Geometry: final body of the model. Coordinates: model frame, mm. A direction names the side the tool comes from. Round coordinates to 2 decimals unless told otherwise and drop trailing zeros. Write each loop counter-clockwise with the first axis right and the second up, starting at its lowest first coordinate (ties: lowest second). Pieces come first, ordered by that corner, then holes. Notation, with made-up numbers: (47, -34.5) -> (99, -34.5) arc R17 cw to (99, -22.5) -> close; hole circle Ø1 at (32, 86). An arc over 180 degrees is marked (long way). Use one line per item in the form item = value. Start each with the question number.
1. Cut plane D-D, the plane y = 4.75. Return the cut outline in (x, z), plus the area to 3 significant figures.
2. Draft query along Z for faces 1 (the face through (-61, 20, 34.421)), 2 (the face through (-50.91, 3.04, 53.85)), 3 (the face through (-47.459, 3, 45)). Return one class per face: pulls with the +Z half, pulls with the -Z half, needs draft (parallel to the pull), parting line crosses it, or undercut.
3. Cut plane A-A, the plane y = 16.5. Return the cut outline in (x, z), plus the area to 3 significant figures.
4. Pin query (flat end, axial travel): pin 1 Ø5 at (x, z) = (-70.5, 39) entering from +Y; pin 2 Ø10 at (y, z) = (16, 50) entering from -X; pin 3 Ø10 at (y, z) = (18.5, 50) entering from +X. Return the tip coordinate at first contact, or that it passes through.
5. Line query: L1, parallel to Z at x = -70, y = 1; L2, parallel to X at y = 15.5, z = 41; L3, parallel to Y at x = -59.5, z = 52.25. Output: solid intervals per line, ascending.
6. Reachability of faces 4 (the face through (-53.459, 15, 45)), 5 (the face through (-70.79, 3.04, 53.11)), 6 (the face through (-60, 12, 46)), 7 (the face through (-66.459, 15, 45)) from +Z, -Z, +X, -X, +Y, -Y: full face, straight path, thin tool, end or side. Return the list, or none.
7. Cut plane B-B, the plane z = 42.75. Return the cut outline in (x, y).
8. Cut plane C-C, the plane x = -61.25. Return the cut outline in (y, z), plus the area to 3 significant figures.
```python
from build123d import *

# Parameters (mm, degrees)
SKETCH_1_W          = 25
SKETCH_1_H          = 25
EXTRUDE_1_DEPTH     = 23
SKETCH_2_W          = 6
SKETCH_2_H          = 25
CUT_EXTRUDE_1_DEPTH = 17
SKETCH_3_R          = 1.5
CUT_EXTRUDE_2_DEPTH = 6
SKETCH_7_W          = 9
SKETCH_7_H          = 9
CUT_EXTRUDE_3_DEPTH = 23
SKETCH_8_R          = 3.1
CUT_EXTRUDE_4_DEPTH = 23


with BuildPart() as part:
    # 草图1 → 凸台-拉伸1 (new body)
    with BuildSketch(Plane(origin=(0, 0, 0), x_dir=(1, 0, 0), z_dir=(0, 1, 0))):
        with Locations((-59.958661712, -44.921006296)):
            Rectangle(SKETCH_1_W, SKETCH_1_H)
    extrude(amount=EXTRUDE_1_DEPTH)

    # 草图2 → 切除-拉伸1 (cut)
    with BuildSketch(Plane(origin=(0, 23, 0), x_dir=(1, 0, 0), z_dir=(0, 1, 0))):
        with Locations((-69.458661712, -44.921006296)):
            Rectangle(SKETCH_2_W, SKETCH_2_H)
        with Locations((-50.458661712, -44.921006296)):
            Rectangle(SKETCH_2_W, SKETCH_2_H)
    extrude(amount=-CUT_EXTRUDE_1_DEPTH, mode=Mode.SUBTRACT)

    # 草图3 → 切除-拉伸2 (cut)
    with BuildSketch(Plane(origin=(0, 6, 0), x_dir=(1, 0, 0), z_dir=(0, 1, 0))):
        with Locations(Location((-69.458661712, -37.421006296, 0), (0, 0, 270))):
            Circle(SKETCH_3_R)
        with Locations(Location((-69.458661712, -52.421006296, 0), (0, 0, 270))):
            Circle(SKETCH_3_R)
    cut_extrude_2 = extrude(amount=-CUT_EXTRUDE_2_DEPTH, mode=Mode.SUBTRACT)

    # 镜向1: 切除-拉伸2 across plane
    add(cut_extrude_2.mirror(Plane.ZY.offset(59.958661712)), mode=Mode.SUBTRACT)

    # 草图7 → 切除-拉伸3 (cut)
    with BuildSketch(Plane.XY.offset(57.421006296)):
        with Locations((-59.958661712, 16.5)):
            Rectangle(SKETCH_7_W, SKETCH_7_H)
    extrude(amount=-CUT_EXTRUDE_3_DEPTH, mode=Mode.SUBTRACT)

    # 草图8 → 切除-拉伸4 (cut)
    with BuildSketch(Plane.XY.offset(34.421006296)):
        with Locations((-59.958661712, 16.5)):
            Circle(SKETCH_8_R)
    extrude(amount=-CUT_EXTRUDE_4_DEPTH, mode=Mode.SUBTRACT)


solid = part.part
```
Outcome:
q1.outline = (-72.46, 32.42) -> (-47.46, 32.42) -> (-47.46, 57.42) -> (-72.46, 57.42) -> close; hole circle Ø3 at (-69.46, 37.42); hole circle Ø3 at (-69.46, 52.42); hole circle Ø3 at (-50.46, 37.42); hole circle Ø3 at (-50.46, 52.42)
q1.area = 597 mm^2
q2.face_1 = pulls with the +Z half
q2.face_2 = undercut
q2.face_3 = needs draft
q3.outline = (-66.46, 32.42) -> (-63.06, 32.42) -> (-63.06, 34.42) -> (-64.46, 34.42) -> (-64.46, 57.42) -> (-66.46, 57.42) -> close; (-56.86, 32.42) -> (-53.46, 32.42) -> (-53.46, 57.42) -> (-55.46, 57.42) -> (-55.46, 34.42) -> (-56.86, 34.42) -> close
q3.area = 106 mm^2
q4.pin_1 = 6
q4.pin_2 = -66.46
q4.pin_3 = -53.46
q5.L1 = 32.42 to 36.02, 38.82 to 51.02, 53.82 to 57.42
q5.L2 = -66.46 to -64.46, -55.46 to -53.46
q5.L3 = 0 to 12, 21 to 23
q6.face_4 = +Z, -Z, +X, +Y
q6.face_5 = +Y, -Y
q6.face_6 = +Z
q6.face_7 = +Z, -Z, -X, +Y
q7.outline = (-72.46, 0) -> (-47.46, 0) -> (-47.46, 6) -> (-53.46, 6) -> (-53.46, 23) -> (-66.46, 23) -> (-66.46, 6) -> (-72.46, 6) -> close; hole (-64.46, 12) -> (-55.46, 12) -> (-55.46, 21) -> (-64.46, 21) -> close
q8.outline = (0, 32.42) -> (13.68, 32.42) -> (13.68, 34.42) -> (12, 34.42) -> (12, 57.42) -> (0, 57.42) -> close; (19.32, 32.42) -> (23, 32.42) -> (23, 57.42) -> (21, 57.42) -> (21, 34.42) -> (19.32, 34.42) -> close
q8.area = 357 mm^2
